```python
from build123d import *

# Parameters (mm, degrees)
BOSS_EXTRUDE1_DEPTH = 2


with BuildPart() as part:
    # Sketch1 → Boss-Extrude1 (new body)
    with BuildSketch(Plane.XY):
        with BuildLine():
            Line((-18, 20), (-15, 20))
            Line((-15, 20), (-15, 22))
            Line((-15, 22), (-5, 22))
            Line((-5, 22), (-5, 20))
            Line((-5, 20), (5, 20))
            Line((5, 20), (5, 22))
            Line((5, 22), (15, 22))
            Line((15, 22), (15, 20))
            Line((15, 20), (18, 20))
            ThreePointArc((18, 20), (11.399404767, 0), (18, -20))
            Line((18, -20), (15, -20))
            Line((15, -20), (15, -22))
            Line((15, -22), (5, -22))
            Line((5, -22), (5, -20))
            Line((5, -20), (-5, -20))
            Line((-5, -20), (-5, -22))
            Line((-5, -22), (-15, -22))
            Line((-15, -22), (-15, -20))
            Line((-15, -20), (-18, -20))
            ThreePointArc((-18, -20), (-11.399404767, 0), (-18, 20))
        make_face()
        with BuildLine():
            Line((-10.520951842, -17), (10.520951842, -17))
            ThreePointArc((10.520951842, -17), (12.193632239, -16.096421584), (12.354914733, -14.20214029))
            ThreePointArc((12.354914733, -14.20214029), (9.399404767, 0), (12.354914733, 14.20214029))
            ThreePointArc((12.354914733, 14.20214029), (12.193632239, 16.096421584), (10.520951842, 17))
            Line((10.520951842, 17), (-10.520951842, 17))
            ThreePointArc((-10.520951842, 17), (-12.193632239, 16.096421584), (-12.354914733, 14.20214029))
            ThreePointArc((-12.354914733, 14.20214029), (-9.399404767, 0), (-12.354914733, -14.20214029))
            ThreePointArc((-12.354914733, -14.20214029), (-12.193632239, -16.096421584), (-10.520951842, -17))
        make_face(mode=Mode.SUBTRACT)
    extrude(amount=BOSS_EXTRUDE1_DEPTH)


solid = part.part
```
Can you work these out from the model? Positions are in its coordinate system, mm. A direction names the side the tool comes from. Coordinates: 2 decimals unless noted, no trailing zeros. Loops run counter-clockwise (first coordinate to the right, second up) from the corner with the lowest first, then second, coordinate; pieces in that order, holes last. Notation, with made-up numbers: (46.25, 74) -> (68.25, 74) arc R30 cw to (68.25, 100) -> close; hole circle Ø11 at (-21.75, 84.5). An arc over 180 degrees is marked (long way). Put each result on its own line as item: value. Start each with the question number.
Q1. I want a section at D-D (y = -18.5). Write out the boundary of the cut face in (x, z).
Q2. I want a section at C-C (y = -5). Write out the boundary of the cut face in (x, z), plus the area to 3 significant figures.
Q3. I want a section at B-B (z = 1.55). Write out the boundary of the cut face in (x, y).
Q4. I want a section at A-A (x = 3). Write out the boundary of the cut face in (y, z), plus the area to 3 significant figures.
Q5. For faces 1 (the face through (17, -20, 1)), 2 (the face through (12.18, -16.12, 0.99)), 3 (the face through (-15, 21, 1)), 4 (the face through (-5, -21, 1)), which set-ups out of +Z, -Z, +X, -X, +Y, -Y let a thin tool reach every point of the face, with its end or its side?
Q6. If I drill on line 1 (Y direction, x = -1.5, z = 0.65); line 2 (Y direction, x = -6, z = 1.7); line 3 (X direction, y = 10, z = 0.9), over which ranges is the centre line in solid material (lowest first)? Write a range as [from, to].
Q7. Thinking about a two-plate mould opening in X: for faces 5 (the face through (0, -20, 1)), 6 (the face through (-17, 20, 1)), 7 (the face through (15, -21, 1)), which applies, pulls with the +X half, pulls with the -X half, needs draft (parallel to the pull), parting line crosses it, or undercut?
Q8. I'm going to push flat-ended pins straight in: P1, Ø0.6, axis at y = -20.5, z = 1, coming from the +X side; P2, Ø0.6, axis at y = -21, z = 1.5, coming from the -X side; P3, Ø0.6, axis at x = -16.5, z = 1, coming from the -Y side. Where does each tip first touch, or does it pass through?
Taken from the geometry:
1. outline: (-16.95, 0) -> (16.95, 0) -> (16.95, 2) -> (-16.95, 2) -> close
2. outline: (-11.77, 0) -> (-9.75, 0) -> (-9.75, 2) -> (-11.77, 2) -> close; (9.75, 0) -> (11.77, 0) -> (11.77, 2) -> (9.75, 2) -> close
2. area: 8.08 mm2
3. outline: (-18, -20) -> (-15, -20) -> (-15, -22) -> (-5, -22) -> (-5, -20) -> (5, -20) -> (5, -22) -> (15, -22) -> (15, -20) -> (18, -20) arc R33.6 cw to (18, 20) -> (15, 20) -> (15, 22) -> (5, 22) -> (5, 20) -> (-5, 20) -> (-5, 22) -> (-15, 22) -> (-15, 20) -> (-18, 20) arc R33.6 cw to start; hole (-12.35, -14.2) arc R2 ccw to (-10.52, -17) -> (10.52, -17) arc R2 ccw to (12.35, -14.2) arc R35.6 cw to (12.35, 14.2) arc R2 ccw to (10.52, 17) -> (-10.52, 17) arc R2 ccw to (-12.35, 14.2) arc R35.6 cw to start
4. outline: (-20, 0) -> (-17, 0) -> (-17, 2) -> (-20, 2) -> close; (17, 0) -> (20, 0) -> (20, 2) -> (17, 2) -> close
4. area: 12.0 mm2
5. face 1: +Z, -Z, +X, -Y
5. face 2: +Z, -Z
5. face 3: +Z, -Z, -X, +Y
5. face 4: +Z, -Z, -Y
6. line 1: y = [-20, -17], [17, 20]
6. line 2: y = [-22, -17], [17, 22]
6. line 3: x = [-12.92, -10.83], [10.83, 12.92]
7. face 5: undercut
7. face 6: needs draft
7. face 7: pulls with the +X half
8. P1: stops at x = 15
8. P2: stops at x = -15
8. P3: stops at y = -20
